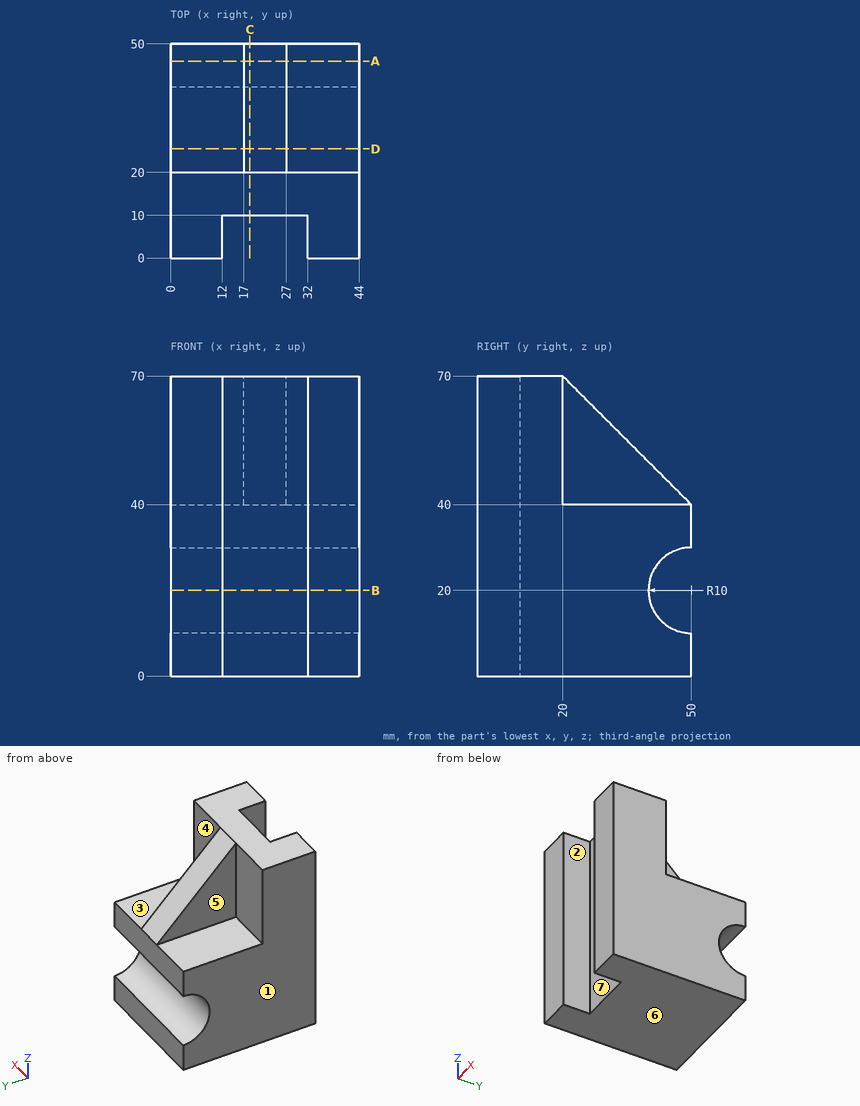
For this review, use the dimensioned drawing (mm, ordinates from the lowest corner) and the shaded views. A direction names the side the tool comes from. Coordinates: 2 decimals unless noted, no trailing zeros. Order: outer loops, then holes, each group sorted by start corner. A loop starts at its lowest first (then second) coordinate and runs counter-clockwise, first axis right, second up. Notation, with made-up numbers: M 79,27.5 L 121,27.5 A12 cw 121,41.5 Z; hole C 85.5,79.25 d6. An arc over 180 degrees is marked long. Answer as a JSON object with one key per item and string values. Group by question number.
1) Add section A-A, the plane y = 46. Write out the cut boundary in (x, z).
2) Add section C-C, the plane x = 18.5. Write out the cut boundary in (y, z), then the cut area to 3 significant figures.
3) Add section B-B, the plane z = 20. Write out the cut boundary in (x, y), then the cut area to 3 significant figures.
4) For pin 1 (12 mm diameter, centred on x = 21.5, y = 36, fed in from +Z); pin 2 (1.5 mm diameter, centred on x = 26.5, y = 25.5, fed in from +Z); pin 3 (5 mm diameter, centred on x = 21.5, y = 28.5, fed in from +Z), all flat-tipped, find the tip position at first contact; note any pin that passes through.
5) Add section D-D, the plane y = 25.5. Write out the cut boundary in (x, z), then the cut area to 4 significant figures.
6) Tool access review of the marked faces 4, 5, 6 and 7: name each direction out of +Z, -Z, +X, -X, +Y, -Y from which nothing blocks a thin tool from reaching the whole face with its end or side.
7) Wall thickness on L1, parallel to X at y = 5, z = 48; L2, parallel to Y at x = 32.5, z = 60.5; L3, parallel to X at y = 42, z = 44: over which ranges is each line inside the solid? List them lowest first.
8) Mouldability with a two-part tool opening along X and no side actions: class the marked faces 1, 2 and 3 as pulls with the +X half, pulls with the -X half, needs draft (parallel to the pull), parting line crosses it, or undercut.
Computed values:
{
 "1": {"outline": "M 0,0 L 44,0 L 44,10.83 L 0,10.83 Z; M 0,29.17 L 44,29.17 L 44,40 L 27,40 L 27,44 L 17,44 L 17,40 L 0,40 Z"},
 "2": {"outline": "M 10,0 L 50,0 L 50,10 A10 cw 50,30 L 50,40 L 20,70 L 10,70 Z", "area": "2,190 mm^2"},
 "3": {"outline": "M 0,0 L 12,0 L 12,10 L 32,10 L 32,0 L 44,0 L 44,40 L 0,40 Z", "area": "1,560 mm^2"},
 "4": {"pin 1": "stops at z = 60", "pin 2": "stops at z = 65.25", "pin 3": "stops at z = 64"},
 "5": {"outline": "M 0,0 L 44,0 L 44,40 L 27,40 L 27,64.5 L 17,64.5 L 17,40 L 0,40 Z", "area": "2,005 mm^2"},
 "6": {"face 4": "+Z, +X, +Y", "face 5": "+Z, -X, +Y", "face 6": "-Z, +X, -X, +Y, -Y", "face 7": "+Z, -Z, -Y"},
 "7": {"L1": "x = 0 to 12, 32 to 44", "L2": "y = 0 to 20", "L3": "x = 17 to 27"},
 "8": {"face 1": "pulls with the -X half", "face 2": "undercut", "face 3": "needs draft"}
}
